Geometry check sheet. Reference: the model listing, model coordinates, mm. A direction names the side the tool comes from. Round coordinates to 2 decimals unless told otherwise and drop trailing zeros. Order: outer loops, then holes, each group sorted by start corner. A loop starts at its lowest first (then second) coordinate and runs counter-clockwise, first axis right, second up. Notation, with made-up numbers: (4.25, 23.25) - (28.25, 23.25) arc R24 cw to (28.25, 44.25) - close; hole circle Ø2 at (44, 43). An arc over 180 degrees is marked (long way). Return JSON: item names as keys, results as strings. Group by question number.
Q1. Sectioned sample at B-B, the plane y = -140.5. Give the number of separate pieces and of enclosed holes in the cut face, then the cut area to 3 significant figures.
Q2. Draft check along X on faces 1 (the flat face through (-1, 0, 2)), 2 (the flat face through (-40, -104, 2)), 3 (the flat face through (-64.222, -128.585, -4.86)). Enter one of: pulls with the +X half, pulls with the -X half, needs draft (parallel to the pull), parting line crosses it, or undercut.
Q3. Sectioned sample at C-C, the plane y = -27. Record the cut outline in (x, z).
Q4. Tool access check on faces 4 (the cylindrical face through (32.706, -122.139, -2.566)), 5 (the flat face through (64, -50, -7)), 6 (the flat face through (40, -104, 2)), 7 (the flat face through (-102.5, -25, 2)). Record the directions out of +Z, -Z, +X, -X, +Y, -Y that give a thin tool (end or side, any length) a straight path to the whole face; none if there is none.
Q5. Sectioned sample at A-A, the plane z = -3. Record the cut outline in (x, y).
Q6. Gauge pin test, flat ends, axial feed: pin 1 Ø8 at (y, z) = (-140, -5) entering from +X; pin 2 Ø5 at (y, z) = (-119, -3) entering from -X; pin 3 Ø4 at (y, z) = (-99, 2) entering from -X; pin 4 Ø12.5 at (x, y) = (-56, -92) entering from -Z. Record the tip position at first contact, or that the pin passes through.
Q7. Material ranges on line 1 along Y through (x, z) = (15, 0.95); line 2 along X through (y, z) = (-195, 2.1); line 3 along X through (y, z) = (-60.5, -4), recorded low to high.
```python
from build123d import *

# Parameters (mm, degrees)
SKETCH019_R     = 2
PAD_DEPTH       = 5
PAD001_DEPTH    = 15
FILLET003_R     = 9
CHAMFER004_SIZE = 2


with BuildPart() as part:
    # Sketch019 → Pad (new body)
    with BuildSketch(Plane.XY):
        Polygon((-102.5, 0), (102.5, 0), (102.5, -50), (27, -205), (-27, -205), (-102.5, -50), align=None)
        with Locations((-87.5, -10)):
            Circle(SKETCH019_R, mode=Mode.SUBTRACT)
        with Locations((87.5, -10)):
            Circle(SKETCH019_R, mode=Mode.SUBTRACT)
        with Locations((-15, -80)):
            Circle(SKETCH019_R, mode=Mode.SUBTRACT)
        with Locations((15, -80)):
            Circle(SKETCH019_R, mode=Mode.SUBTRACT)
        with Locations((-15, -195)):
            Circle(SKETCH019_R, mode=Mode.SUBTRACT)
        with Locations((15, -195)):
            Circle(SKETCH019_R, mode=Mode.SUBTRACT)
        Polygon((-78.508698, -65), (-40, -65), (-40, -144.057592), align=None, mode=Mode.SUBTRACT)
        Polygon((78.508698, -65), (40, -65), (40, -144.057592), align=None, mode=Mode.SUBTRACT)
    extrude(amount=PAD_DEPTH)

    # Sketch020 → Pad001 (join)
    with BuildSketch(Plane.XY):
        Polygon((-25, -50), (-25, -205), (-27, -205), (-102.5, -50), align=None)
        Polygon((-30, -187.423171), (-30, -55), (-94.502899, -55), align=None, mode=Mode.SUBTRACT)
        Polygon((25, -50), (25, -205), (27, -205), (102.5, -50), align=None)
        Polygon((94.502899, -55), (30, -55), (30, -187.423171), align=None, mode=Mode.SUBTRACT)
    extrude(amount=-PAD001_DEPTH)

    # Fillet003
    fillet003_edges = [part.edges().sort_by_distance(p)[0] for p in [
        (30, -121.211585, 0),
        (-62.25145, -55, 0),
        (-62.25145, -121.211585, 0),
        (62.25145, -55, 0),
        (62.25145, -121.211585, 0),
        (-30, -121.211585, 0),
    ]]
    fillet(fillet003_edges, radius=FILLET003_R)

    # Chamfer004
    chamfer004_edges = [part.edges().sort_by_distance(p)[0] for p in [
        (-89.5, -10, 5),
        (85.5, -10, 5),
        (-17, -80, 5),
        (13, -80, 5),
        (-17, -195, 5),
        (13, -195, 5),
    ]]
    chamfer(chamfer004_edges, length=CHAMFER004_SIZE)


solid = part.part
```
Reply:
{
 "1": {"separate pieces": "3", "enclosed holes": "0", "area": "957 mm^2"},
 "2": {"face 1": "needs draft", "face 2": "undercut", "face 3": "pulls with the -X half"},
 "3": {"outline": "(-102.5, 0) - (102.5, 0) - (102.5, 5) - (-102.5, 5) - close"},
 "4": {"face 4": "-Z", "face 5": "-Z, +X, -X, +Y", "face 6": "+Z, -Z", "face 7": "+Z, -Z, -X, +Y, -Y"},
 "5": {"outline": "(-102.5, -50) - (-27, -205) - (-25, -205) - (-25, -50) - close; (25, -205) - (27, -205) - (102.5, -50) - (25, -50) - close; hole (-90.84, -57.29) - (-32.29, -177.48) - (-32.29, -57.29) - close; hole (32.29, -177.48) - (90.84, -57.29) - (32.29, -57.29) - close"},
 "6": {"pin 1": "x = 60.61", "pin 2": "x = -70.11", "pin 3": "x = -79.61", "pin 4": "through"},
 "7": {"line 1": "-205 to -197, -193 to -82, -78 to 0", "line 2": "-31.87 to -17, -13 to 13, 17 to 31.87", "line 3": "-97.39 to -90.14, -31.52 to -25, 25 to 31.52, 90.14 to 97.39"}
}
